Design review of the part built by this model. Coordinates are the model's own, in mm. A direction names the side the tool comes from. Give positions to 0.01 mm unless a question says otherwise; leave off trailing zeros. Write each loop counter-clockwise with the first axis right and the second up, starting at its lowest first coordinate (ties: lowest second). Pieces come first, ordered by that corner, then holes. Notation, with made-up numbers: (87, 0.25) -> (99, 0.25) arc R15 ccw to (99, 21.25) -> close; hole circle Ø11 at (26, 53.25). An arc over 180 degrees is marked (long way). Answer as a JSON object with one key per item and string values.
```python
from build123d import *

# Parameters (mm, degrees)
SKETCH1_R           = 4.5
BOSS_EXTRUDE1_DEPTH = 4.3
SKETCH2_R           = 3
BOSS_EXTRUDE2_DEPTH = 2
SKETCH3_R           = 1.55
CUT_EXTRUDE1_DEPTH  = 9.954886934
BOSS_EXTRUDE3_START = 2.5
SKETCH4_R           = 4.5
SKETCH4_R_2         = 3.8
BOSS_EXTRUDE3_DEPTH = 2.5
CUT_EXTRUDE2_DEPTH  = 9.954886934


with BuildPart() as part:
    # Sketch1 → Boss-Extrude1 (new body)
    with BuildSketch(Plane(origin=(0, 0, 0), x_dir=(1, 0, 0), z_dir=(0, 1, 0))):
        with Locations(Location((0, 0, 0), (0, 0, 90))):
            Circle(SKETCH1_R)
    extrude(amount=BOSS_EXTRUDE1_DEPTH)

    # Sketch2 → Boss-Extrude2 (add)
    with BuildSketch(Plane(origin=(0, 4.3, 0), x_dir=(1, 0, 0), z_dir=(0, 1, 0))):
        with Locations(Location((0, 0, 0), (0, 0, 270))):
            Circle(SKETCH2_R)
    extrude(amount=BOSS_EXTRUDE2_DEPTH)

    # Sketch3 → Cut-Extrude1 (cut, through all)
    with BuildSketch(Plane(origin=(0, 6.3, 0), x_dir=(1, 0, 0), z_dir=(0, 1, 0))):
        with Locations(Location((0, 0, 0), (0, 0, 270))):
            Circle(SKETCH3_R)
    extrude(amount=-CUT_EXTRUDE1_DEPTH, mode=Mode.SUBTRACT)

    # Sketch4 → Boss-Extrude3 (add)
    with BuildSketch(Plane.XZ.offset(BOSS_EXTRUDE3_START)):
        with Locations(Location((0, 0, 0), (0, 0, 270))):
            Circle(SKETCH4_R)
        with Locations(Location((0, 0, 0), (0, 0, 270))):
            Circle(SKETCH4_R_2, mode=Mode.SUBTRACT)
    extrude(amount=-BOSS_EXTRUDE3_DEPTH)

    # Sketch5 → Cut-Extrude2 (cut, through all)
    with BuildSketch(Plane.XZ):
        Polygon((0, 0), (0, 5.809318517), (6.55644872, 5.809318517), (6.55644872, 1.25), (2.958025702, 1.25), (2.958025702, -1.25), (6.55644872, -1.25), (6.55644872, -5.809318517), (0, -5.809318517), align=None)
    extrude(amount=CUT_EXTRUDE2_DEPTH, mode=Mode.SUBTRACT)


solid = part.part
```
(1) We need section A-A, the plane z = 0. State the section outline as (x, y) points, then the cut area to 3 significant figures.
Here are the results:
{"outline": "(-4.5, -2.5) -> (-3.8, -2.5) -> (-3.8, 0) -> (-1.55, 0) -> (-1.55, 6.3) -> (-3, 6.3) -> (-3, 4.3) -> (-4.5, 4.3) -> close; (1.55, 0) -> (3.8, 0) -> (3.8, -2.5) -> (4.5, -2.5) -> (4.5, 4.3) -> (3, 4.3) -> (3, 6.3) -> (1.55, 6.3) -> close", "area": "34.7 mm²"}
(2) Clearance check with flat-ended pins moving along their axes: pin 1 (3 mm diameter, centred on x = -3, y = 5, fed in from -Z); pin 2 (0.6 mm diameter, centred on x = 4, y = -1, fed in from +Z); pin 3 (0.6 mm diameter, centred on y = -1.5, z = -4, fed in from +X). State where each tip first meets the part, or that it passes through.
Here are the results:
{"pin 1": "stops at z = -4.18", "pin 2": "stops at z = 1.25", "pin 3": "stops at x = 0"}
(3) We need section B-B, the plane y = -1. State the section outline as (x, z) points.
Here are the results:
{"outline": "(0, -4.5) -> (0, -3.8) arc R3.8 cw to (0, 3.8) -> (0, 4.5) arc R4.5 ccw to start; (3.59, -1.25) -> (4.32, -1.25) arc R4.5 ccw to (4.32, 1.25) -> (3.59, 1.25) arc R3.8 cw to start"}
(4) We need section D-D, the plane y = 1.5. State the section outline as (x, z) points, then the cut area to 3 significant figures.
Here are the results:
{"outline": "circle Ø9 at (0, 0); hole circle Ø3.1 at (0, 0)", "area": "56.1 mm²"}
(5) For line 1 along X through (y, z) = (2, 0); line 2 along X through (y, z) = (4.75, 0); line 3 along Y through (x, z) = (-0.5, 4), list the stretches that pass through material, from the lowest coordinate up.
Here are the results:
{"line 1": "x = -4.5 to -1.55, 1.55 to 4.5", "line 2": "x = -3 to -1.55, 1.55 to 3", "line 3": "y = -2.5 to 4.3"}
(6) For faces 4 (the flat face through (-4, -2.5, 0)), 5 (the flat face through (3, 4.3, -1)), 6 (the cylindrical face through (-3.8, -1.3, 0.1)), list the 3-axis set-ups (+Z, -Z, +X, -X, +Y, -Y) from which the entire face can be reached by the end or side of a thin tool; tool diameter is ignored.
Here are the results:
{"face 4": "+Z, -Z, +X, -X, -Y", "face 5": "+Y", "face 6": "-Y"}
(7) The part is to be moulded in two halves that separate along Z. For faces 1 (the cylindrical face through (0.466, 3.194, 1.478)), 2 (the cylindrical face through (0.9, 5.29, 2.86)), 3 (the flat face through (4, -2.5, 0)), say which applies: +Z half, -Z half, draft (parallel to the pull), parting line (faces both ways), or undercut.
Here are the results:
{"face 1": "undercut", "face 2": "parting line", "face 3": "draft"}
(8) We need section C-C, the plane x = -0.5. State the section outline as (y, z) points.
Here are the results:
{"outline": "(-2.5, -4.47) -> (4.3, -4.47) -> (4.3, -2.96) -> (6.3, -2.96) -> (6.3, -1.47) -> (0, -1.47) -> (0, -3.77) -> (-2.5, -3.77) -> close; (-2.5, 3.77) -> (0, 3.77) -> (0, 1.47) -> (6.3, 1.47) -> (6.3, 2.96) -> (4.3, 2.96) -> (4.3, 4.47) -> (-2.5, 4.47) -> close"}
